Read the model definition and answer for the solid it produces. Units are mm, in the model's axes. Face numbers are marked on the shaded views. A direction names the side the tool comes from. Round coordinates to 2 decimals unless told otherwise and drop trailing zeros. Loops run counter-clockwise (first coordinate to the right, second up) from the corner with the lowest first, then second, coordinate; pieces in that order, holes last. Notation, with made-up numbers: M -4.5,48.5 L 16.5,48.5 A9 ccw 16.5,55.5 Z; hole C 66,-1 d1. An arc over 180 degrees is marked long. Write each question's results on one line, items separated by ' | '.
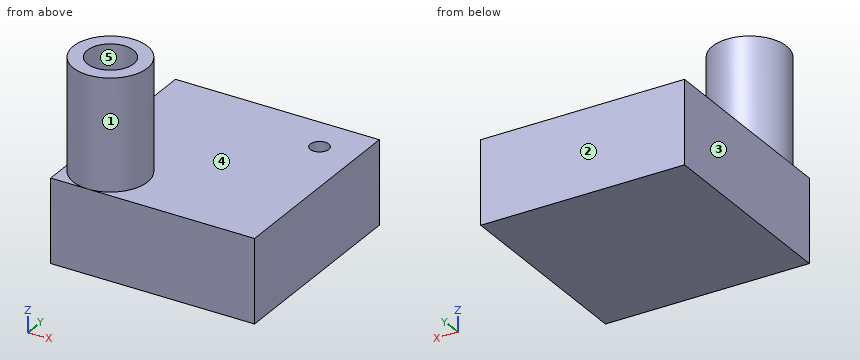
from build123d import *

# Parameters (mm, degrees)
TORUS_R           = 3.5
CYLINDER002_R     = 1
CYLINDER002_DEPTH = 10
CYLINDER_R        = 2.5
CYLINDER_DEPTH    = 17
CYLINDER001_R     = 4
CYLINDER001_DEPTH = 17
BOX_W             = 22
BOX_H             = 22
BOX_DEPTH         = 9


with BuildPart() as torus:
    # Torus → Torus (revolve)
    with BuildSketch(Plane(origin=(3, 3, 4), x_dir=(1, 0, 0), z_dir=(0, -1, 0))):
        with Locations((7, 0)):
            Circle(TORUS_R)
    revolve(axis=Axis((3, 3, 4), (0, 0, 1)))


with BuildPart() as cylinder002:
    # Cylinder002 → Cylinder002 (new body)
    with BuildSketch(Plane(origin=(10, 10, 7), x_dir=(1, 0, 0), z_dir=(0, 0, 1))):
        Circle(CYLINDER002_R)
    extrude(amount=CYLINDER002_DEPTH)


with BuildPart() as fusion:
    # Cylinder → Cylinder (new body)
    with BuildSketch(Plane(origin=(-4, -4, 4), x_dir=(1, 0, 0), z_dir=(0, 0, 1))):
        Circle(CYLINDER_R)
    extrude(amount=CYLINDER_DEPTH)

    # Fusion: union Torus, Cylinder002
    add(torus.part)
    add(cylinder002.part)


with BuildPart() as cylinder001:
    # Cylinder001 → Cylinder001 (new body)
    with BuildSketch(Plane(origin=(-4, -4, 4), x_dir=(1, 0, 0), z_dir=(0, 0, 1))):
        Circle(CYLINDER001_R)
    extrude(amount=CYLINDER001_DEPTH)


with BuildPart() as cut:
    # Box → Box (new body)
    with BuildSketch(Plane(origin=(-8, -8, 0), x_dir=(1, 0, 0), z_dir=(0, 0, 1))):
        with Locations((11, 11)):
            Rectangle(BOX_W, BOX_H)
    extrude(amount=BOX_DEPTH)

    # Fusion001: union Cylinder001
    add(cylinder001.part)

    # Cut: cut Fusion
    add(fusion.part, mode=Mode.SUBTRACT)


solid = cut.part
Item 1: The part is cut by section A-A (z = 6.5). Determine the outline of the cut face in (x, y), plus the area to 3 significant figures.
Outcome:
outline: M -8,-8 L 14,-8 L 14,14 L -8,14 Z; C 3,3 d9.1; hole M -5.15,-1.78 A2.5 ccw long -1.78,-5.15 A9.45 ccw long Z | area: 256 mm2
Item 2: Flat-ended cylindrical pins translate along their axes: pin 1 (1 mm diameter, centred on x = 10, y = 10, fed in from +Z); pin 2 (1.5 mm diameter, centred on x = 2.5, y = -0.5, fed in from +Z); pin 3 (1.2 mm diameter, centred on x = -5.5, y = -4.5, fed in from +Z). Find the tip coordinate at first contact, or state that the pin passes through.
Outcome:
pin 1: stops at z = 7 | pin 2: stops at z = 9 | pin 3: stops at z = 4
Item 3: The part is cut by section C-C (z = 12). Determine the outline of the cut face in (x, y).
Outcome:
outline: C -4,-4 d8; hole C -4,-4 d5
Item 4: Straight lines are drawn through the part: line 1 (Z direction, x = -4, y = 2.5); line 2 (Y direction, x = 10, z = 7.85); line 3 (Y direction, x = 1.5, z = 5.25). For each, find the intervals that lie inside material, in ascending order.
Outcome:
line 1: z = 0 to 0.5, 7.5 to 9 | line 2: y = -8 to 9, 11 to 14 | line 3: y = -8 to -7.16, -0.42 to 6.42, 13.16 to 14
Item 5: The part is cut by section B-B (z = 2.5). Determine the outline of the cut face in (x, y), plus the area to 3 significant figures.
Outcome:
outline: M -8,-8 L 14,-8 L 14,14 L -8,14 Z; C 3,3 d7.68; hole C 3,3 d20.32 | area: 206 mm2
Item 6: The mould has two halves that part along X. Classify the marked faces 3, 4 and 5: pulls with the +X half, pulls with the -X half, needs draft (parallel to the pull), parting line crosses it, or undercut.
Outcome:
face 3: pulls with the -X half | face 4: needs draft | face 5: undercut
Item 7: For the marked faces 1 and 2, determine the directions among +Z, -Z, +X, -X, +Y, -Y from which every point of the face is accessible in a straight line to the end or side of a thin tool.
Outcome:
face 1: +Z | face 2: +Z, -Z, +X, -X, +Y
Item 8: The part is cut by section D-D (y = 0.75). State how many separate pieces and enclosed holes the cut face has, plus the area to 3 significant figures.
Outcome:
separate pieces: 1 | enclosed holes: 2 | area: 115 mm2
